Check sheet for the modelled part. Datum: model origin and axes. Units: mm. A direction names the side the tool comes from. Coordinates: 2 decimals unless noted, no trailing zeros. Write each loop counter-clockwise with the first axis right and the second up, starting at its lowest first coordinate (ties: lowest second). Pieces come first, ordered by that corner, then holes. Notation, with made-up numbers: (62, 12.5) - (97, 12.5) arc R26 cw to (97, 30.5) - close; hole circle Ø5 at (-12.5, 35.5). An arc over 180 degrees is marked (long way). Write each question's results on one line, items separated by ' | '.
from build123d import *

# Parameters (mm, degrees)
SKETCH1_R           = 13.5
SKETCH1_R_2         = 12.5
BOSS_EXTRUDE1_DEPTH = 175
SKETCH3_W           = 50
SKETCH3_H           = 3
CUT_EXTRUDE1_START  = -40.25
CUT_EXTRUDE1_DEPTH  = 40.25
CUT_EXTRUDE2_REACH  = 181.854
SKETCH5_R           = 12.5


# Read off the part's stored shape, not the designer's step: Cut-Extrude1
with BuildPart() as part:
    # Sketch1 → Boss-Extrude1 (new body)
    with BuildSketch(Plane(origin=(0, 0, 0), x_dir=(1, 0, 0), z_dir=(0, 1, 0))):
        with Locations(Location((0, 0, 0), (0, 0, 270))):
            Circle(SKETCH1_R)
        with Locations(Location((0, 0, 0), (0, 0, 270))):
            Circle(SKETCH1_R_2, mode=Mode.SUBTRACT)
    extrude(amount=BOSS_EXTRUDE1_DEPTH)

    # Sweep1: sweep along a path in Sketch2
    with BuildLine(Plane.XY) as sweep1_path:
        Line((38.75, -147), (38.75, -47))
        Line((38.75, -47), (13.5, 3))
        Line((13.5, 3), (0, 3))
    # Sketch3 → Sweep1 (sweep)
    with BuildSketch(Plane(origin=(0, 0, 0), x_dir=(0, 0, -1), z_dir=(1, 0, 0))):
        with Locations((0, 3)):
            Rectangle(SKETCH3_W, SKETCH3_H)
    sweep1 = sweep(path=sweep1_path.line, transition=Transition.RIGHT)

    # Cut-Extrude1 outline → Cut-Extrude1 (cut)
    with BuildSketch(Plane(origin=(40.25, 0, 0), x_dir=(0, 0, -1), z_dir=(1, 0, 0)).offset(CUT_EXTRUDE1_START)):
        with BuildLine():
            Line((25, -147), (25, 4.5))
            Line((25, 4.5), (17.5, -130.560717777))
            ThreePointArc((17.5, -130.560717777), (14.3396304, -140.591919101), (6, -147))
            Line((6, -147), (25, -147))
        make_face()
        with BuildLine():
            Line((-25, -147), (-6, -147))
            ThreePointArc((-6, -147), (-14.3396304, -140.591919101), (-17.5, -130.560717777))
            Line((-17.5, -130.560717777), (-25, 4.5))
            Line((-25, 4.5), (-25, -147))
        make_face()
        with BuildLine():
            Line((-6, -147), (6, -147))
            Line((6, -147), (6, -130.560717777))
            ThreePointArc((6, -130.560717777), (0, -124.560717777), (-6, -130.560717777))
            Line((-6, -130.560717777), (-6, -147))
        make_face()
    cut_extrude1 = extrude(amount=CUT_EXTRUDE1_DEPTH, mode=Mode.SUBTRACT)

    # Mirror1: Sweep1, Cut-Extrude1 across plane
    add(sweep1.mirror(Plane(origin=(0, 0, 0), x_dir=(0, 0, 1), z_dir=(1, 0, 0))))
    add(cut_extrude1.mirror(Plane(origin=(0, 0, 0), x_dir=(0, 0, 1), z_dir=(1, 0, 0))), mode=Mode.SUBTRACT)

    # Sketch5 → Cut-Extrude2 (cut, up to next)
    with BuildSketch(Plane.XZ.offset(-1.5), mode=Mode.PRIVATE) as cut_extrude2_sk1:
        with Locations(Location((0, 0, 0), (0, 0, 90))):
            Circle(SKETCH5_R)
    cut_extrude2_tool1 = extrude(cut_extrude2_sk1.sketch, amount=-CUT_EXTRUDE2_REACH, mode=Mode.PRIVATE) & part.part
    add(cut_extrude2_tool1.solids().sort_by_distance((0, 1.5, 0))[0], mode=Mode.SUBTRACT)


solid = part.part
1. Material ranges on L1, parallel to X at y = 72.5, z = 0; L2, parallel to X at y = -88.5, z = 0; L3, parallel to Y at x = -9, z = -9, recorded low to high. Write a range as [from, to].
Values follow:
L1: x = [-13.5, -12.5], [12.5, 13.5] | L2: x = [-40.25, -37.25], [37.25, 40.25] | L3: y = [0, 175]
2. Go/stop test with flat-tipped pins: pin 1 (0.9 mm diameter, centred on x = -38.5, y = -142.5, fed in from +Z); pin 2 (8 mm diameter, centred on x = 10.5, z = -12.5, fed in from +Y); pin 3 (2.5 mm diameter, centred on x = 38, y = -142.5, fed in from +Z); pin 4 (4 mm diameter, centred on x = 27, z = 18, fed in from -Y). Record where each tip stops, or that it passes through.
Values follow:
pin 1: stops at z = 13.2 | pin 2: stops at y = 175 | pin 3: stops at z = 13.86 | pin 4: stops at y = -31.02
3. Sectioned sample at B-B (z = -9). Record the cut outline in (x, y), then the cut area to 3 significant figures.
Values follow:
outline: (-40.25, -145.57) - (-37.25, -145.57) - (-37.25, -47.36) - (-12.58, 1.5) - (-10.06, 1.5) - (-10.06, 0) - (-8.67, 0) - (-8.67, 175) - (-10.06, 175) - (-10.06, 4.5) - (-14.42, 4.5) - (-40.25, -46.64) - close; (8.67, 0) - (10.06, 0) - (10.06, 1.5) - (12.58, 1.5) - (37.25, -47.36) - (37.25, -145.57) - (40.25, -145.57) - (40.25, -46.64) - (14.42, 4.5) - (10.06, 4.5) - (10.06, 175) - (8.67, 175) - close | area: 1,430 mm^2
4. Sectioned sample at C-C (y = -73). Record the cut outline in (x, z).
Values follow:
outline: (-40.25, -20.7) - (-37.25, -20.7) - (-37.25, 20.7) - (-40.25, 20.7) - close; (37.25, -20.7) - (40.25, -20.7) - (40.25, 20.7) - (37.25, 20.7) - close
5. Sectioned sample at D-D (y = 64). Record the cut outline in (x, z), then the cut area to 3 significant figures.
Values follow:
outline: circle Ø27 at (0, 0); hole circle Ø25 at (0, 0) | area: 81.7 mm^2
6. Draft check along X on faces 1 (the flat face through (-27.156, -20.713, -0.35)), 2 (the cylindrical face through (-13.18, 88.56, -2.93)), 3 (the flat face through (-9, 175, 9)), 4 (the cylindrical face through (-0.267, 0.74, 13.497)). Enter one of: pulls with the +X half, pulls with the -X half, needs draft (parallel to the pull), parting line crosses it, or undercut.
Values follow:
face 1: pulls with the -X half | face 2: parting line crosses it | face 3: needs draft | face 4: undercut
7. Access from +Z, -Z, +X, -X, +Y, -Y to the whole of each face (thin tool, end or side, straight path). Record for faces 5 (the cylindrical face through (-38.729, -124.562, -0.132)), 6 (the flat face through (0, 1.5, 17)), 7 (the flat face through (13, 4.5, -6)), 8 (the flat face through (-9, 0, -9)).
Values follow:
face 5: +X, -X, -Y | face 6: +Z, -Y | face 7: +Y | face 8: +Z, -Z, -Y
8. Sectioned sample at A-A (x = 0). Record the cut outline in (y, z).
Values follow:
outline: (0, -13.5) - (1.5, -13.5) - (1.5, -24.83) - (4.5, -25) - (4.5, -13.5) - (175, -13.5) - (175, -12.5) - (0, -12.5) - close; (0, 12.5) - (175, 12.5) - (175, 13.5) - (4.5, 13.5) - (4.5, 25) - (1.5, 24.83) - (1.5, 13.5) - (0, 13.5) - close
